```python
from build123d import *

# Parameters (mm, degrees)
F0_W     = 711.2
F0_H     = 635
F0_W_2   = 266.7
F0_H_2   = 241.3
F0_W_3   = 558.8
F0_R     = 12.7
F1_DEPTH = 241.3
F2_DEPTH = 152.4
F3_DEPTH = 6.35
F4_DEPTH = 19.05


with BuildPart() as f1:
    # F0 (on Front) → F1 (new body)
    with BuildSketch(Plane.XZ):
        with Locations((355.6, 317.5)):
            Rectangle(F0_W, F0_H)
        with Locations((209.55, 196.85)):
            Rectangle(F0_W_2, F0_H_2, mode=Mode.SUBTRACT)
        with Locations((501.65, 196.85)):
            Rectangle(F0_W_2, F0_H_2, mode=Mode.SUBTRACT)
        with Locations((355.6, 463.55)):
            Rectangle(F0_W_3, F0_H_2, mode=Mode.SUBTRACT)
        Polygon((-25.4, 635), (0, 635), (711.2, 635), (736.6, 635), (736.6, 660.4), (-25.4, 660.4), align=None)
        with Locations((209.55, 196.85)):
            Rectangle(F0_W_2, F0_H_2)
        with Locations((292.1, 196.85)):
            Circle(F0_R, mode=Mode.SUBTRACT)
        with Locations((501.65, 196.85)):
            Rectangle(F0_W_2, F0_H_2)
        with Locations((419.1, 196.85)):
            Circle(F0_R, mode=Mode.SUBTRACT)
        with Locations((419.1, 196.85)):
            Circle(F0_R)
        with Locations((292.1, 196.85)):
            Circle(F0_R)
        with Locations((355.6, 463.55)):
            Rectangle(F0_W_3, F0_H_2)
    extrude(amount=-F1_DEPTH)

    # F0 (on Front) → F2 (cut)
    with BuildSketch(Plane.XZ):
        with Locations((355.6, 463.55)):
            Rectangle(F0_W_3, F0_H_2)
    extrude(amount=-F2_DEPTH, mode=Mode.SUBTRACT)

    # F0 (on Front) → F3 (join)
    with BuildSketch(Plane.XZ):
        with Locations((209.55, 196.85)):
            Rectangle(F0_W_2, F0_H_2)
        with Locations((292.1, 196.85)):
            Circle(F0_R, mode=Mode.SUBTRACT)
        with Locations((501.65, 196.85)):
            Rectangle(F0_W_2, F0_H_2)
        with Locations((419.1, 196.85)):
            Circle(F0_R, mode=Mode.SUBTRACT)
        with Locations((419.1, 196.85)):
            Circle(F0_R)
        with Locations((292.1, 196.85)):
            Circle(F0_R)
    extrude(amount=F3_DEPTH)

    # F0 (on Front) → F4 (join)
    with BuildSketch(Plane.XZ):
        with Locations((419.1, 196.85)):
            Circle(F0_R)
        with Locations((292.1, 196.85)):
            Circle(F0_R)
    extrude(amount=F4_DEPTH)


solid = f1.part
```
Geometry: final body of the model. Coordinates: model frame, mm. A direction names the side the tool comes from. Round coordinates to 2 decimals unless told otherwise and drop trailing zeros. Write each loop counter-clockwise with the first axis right and the second up, starting at its lowest first coordinate (ties: lowest second). Pieces come first, ordered by that corner, then holes. Notation, with made-up numbers: M -13,66 L 20,66 A8 ccw 20,77 Z; hole C 52.25,65 d5. An arc over 180 degrees is marked long. Answer in a Markdown table with one row per item. Add a question column.
(1) Draft query along X for faces 6 (the face through (406.412, -12.611, 197.408)), 7 (the face through (76.2, 75, 462)), 8 (the face through (-25.4, 119, 648)), 9 (the face through (736.6, 119, 648)). Return one class per face: pulls with the +X half, pulls with the -X half, needs draft (parallel to the pull), parting line crosses it, or undercut.
(2) Cut plane B-B, the plane z = 533. Return the cut outline in (x, y), then the cut area to 3 significant figures.
(3) Cut plane A-A, the plane y = 62. Return the cut outline in (x, z), then the cut area to 3 significant figures.
(4) Reachability of faces 1 (the face through (724, 119, 635)), 2 (the face through (352, 75, 342.9)), 3 (the face through (0, 119, 313)), 4 (the face through (419, -19.05, 197)), 5 (the face through (350, 241.3, 335)) from +Z, -Z, +X, -X, +Y, -Y: full face, straight path, thin tool, end or side. Return the list, or none.
(5) Contact query for flat-ended pins moving along their axis: pin 1 (7 mm diameter, centred on y = -4.5, z = 221, fed in from +X); pin 2 (20.5 mm diameter, centred on x = -14.5, y = 118, fed in from -Z); pin 3 (3 mm diameter, centred on x = 618, z = 519, fed in from -Y). Output: stop coordinate, or through.
(6) Ray query, L1, parallel to Z at x = 110.5, y = 120; L2, parallel to Y at x = 612, z = 412.5; L3, parallel to X at y = 31.5, z = 435.5. Return the intervals inside material, ascending.
(7) Cut plane D-D, the plane y = 224. Return the cut outline in (x, z), then the cut area to 3 significant figures.
(8) Cut plane C-C, the plane x = 292.1. Return the cut outline in (y, z).
Established:
| question | item | result |
|---|---|---|
| 1 | face 6 | undercut |
| 1 | face 7 | undercut |
| 1 | face 8 | pulls with the -X half |
| 1 | face 9 | pulls with the +X half |
| 2 | outline | M 0,0 L 76.2,0 L 76.2,152.4 L 635,152.4 L 635,0 L 711.2,0 L 711.2,241.3 L 0,241.3 Z |
| 2 | area | 86,500 mm² |
| 3 | outline | M -25.4,635 L 0,635 L 0,0 L 711.2,0 L 711.2,635 L 736.6,635 L 736.6,660.4 L -25.4,660.4 Z; hole M 76.2,342.9 L 635,342.9 L 635,584.2 L 76.2,584.2 Z |
| 3 | area | 336,000 mm² |
| 4 | face 1 | -Z, +X, +Y, -Y |
| 4 | face 2 | -Y |
| 4 | face 3 | -Z, -X, +Y, -Y |
| 4 | face 4 | +Z, -Z, +X, -X, -Y |
| 4 | face 5 | +Z, -Z, +X, -X, +Y |
| 5 | pin 1 | x = 635 |
| 5 | pin 2 | z = 635 |
| 5 | pin 3 | y = 152.4 |
| 6 | L1 | 0 to 342.9, 584.2 to 660.4 |
| 6 | L2 | 152.4 to 241.3 |
| 6 | L3 | 0 to 76.2, 635 to 711.2 |
| 7 | outline | M -25.4,635 L 0,635 L 0,0 L 711.2,0 L 711.2,635 L 736.6,635 L 736.6,660.4 L -25.4,660.4 Z |
| 7 | area | 471,000 mm² |
| 8 | outline | M -19.05,184.15 L -6.35,184.15 L -6.35,76.2 L 0,76.2 L 0,0 L 241.3,0 L 241.3,660.4 L 0,660.4 L 0,584.2 L 152.4,584.2 L 152.4,342.9 L 0,342.9 L 0,317.5 L -6.35,317.5 L -6.35,209.55 L -19.05,209.55 Z |
